```python
from build123d import *

# Parameters (mm, degrees)
F0_R     = 11
F1_DEPTH = 25


with BuildPart() as f1:
    # F0 (on Top) → F1 (new body)
    with BuildSketch(Plane.XY):
        with BuildLine():
            ThreePointArc((12.5, -8.291562), (40, 0), (12.5, 8.291562))
            ThreePointArc((12.5, 8.291562), (10.606602, 10.606602), (8.291562, 12.5))
            ThreePointArc((8.291562, 12.5), (0, 40), (-8.291562, 12.5))
            ThreePointArc((-8.291562, 12.5), (-10.606602, 10.606602), (-12.5, 8.291562))
            ThreePointArc((-12.5, 8.291562), (-40, 0), (-12.5, -8.291562))
            ThreePointArc((-12.5, -8.291562), (-10.606602, -10.606602), (-8.291562, -12.5))
            ThreePointArc((-8.291562, -12.5), (0, -40), (8.291562, -12.5))
            ThreePointArc((8.291562, -12.5), (10.606602, -10.606602), (12.5, -8.291562))
        make_face()
        with Locations((0, -25)):
            Circle(F0_R, mode=Mode.SUBTRACT)
        with Locations((-25, 0)):
            Circle(F0_R, mode=Mode.SUBTRACT)
        Circle(F0_R, mode=Mode.SUBTRACT)
        with Locations((25, 0)):
            Circle(F0_R, mode=Mode.SUBTRACT)
        with Locations((0, 25)):
            Circle(F0_R, mode=Mode.SUBTRACT)
    extrude(amount=F1_DEPTH)


solid = f1.part
```
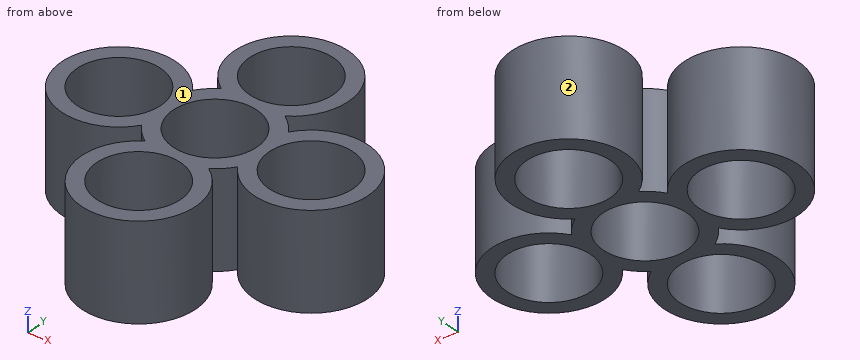
Geometry: final body of the model. Coordinates: model frame, mm. Face numbers are marked on the shaded views. Round coordinates to 2 decimals unless told otherwise and drop trailing zeros. Write each loop counter-clockwise with the first axis right and the second up, starting at its lowest first coordinate (ties: lowest second). Pieces come first, ordered by that corner, then holes. Notation, with made-up numbers: (-20.5, 77.25) -> (29.5, 77.25) arc R18 ccw to (29.5, 101.25) -> close; hole circle Ø8 at (7, 19). An arc over 180 degrees is marked (long way). Use CSV: the item, a comma, the result in double quotes. Start each with the question number.
Q1. Line query: L1, parallel to Y at x = 0, z = 6.5; L2, parallel to X at y = 0.5, z = 11; L3, parallel to Y at x = -25, z = 13.75. Output: solid intervals per line, ascending.
Q2. Section A-A (x = 0). Return loops of the section in (y, z), plus the area to 3 significant figures.
Q3. Section C-C (z = 19). Return loops of the section in (x, y), plus the area to 3 significant figures.
Q4. Section B-B (y = 25). Return loops of the section in (x, z), plus the area to 3 significant figures.
Q5. First-contact query: pin 1 Ø10 at (y, z) = (-21.5, 4.5) entering from +X; pin 2 Ø4 at (x, z) = (-28, 20.5) entering from -Y; pin 3 Ø1.5 at (y, z) = (-13.5, 19.5) entering from +X. Flat tips, straight axial feed; report the tip coordinate or a pass-through.
Q6. Pull-direction query (Y, two-part tool) for the marked faces 1 and 2; classes: pulls with the +Y half, pulls with the -Y half, needs draft (parallel to the pull), parting line crosses it, or undercut.
Result sheet:
1,L1,"-40 to -36, -14 to -11, 11 to 14, 36 to 40"
1,L2,"-39.99 to -35.99, -14.01 to -10.99, 10.99 to 14.01, 35.99 to 39.99"
1,L3,"-15 to -11, 11 to 15"
2,outline,"(-40, 0) -> (-36, 0) -> (-36, 25) -> (-40, 25) -> close; (-14, 0) -> (-11, 0) -> (-11, 25) -> (-14, 25) -> close; (11, 0) -> (14, 0) -> (14, 25) -> (11, 25) -> close; (36, 0) -> (40, 0) -> (40, 25) -> (36, 25) -> close"
2,area,"350 mm²"
3,outline,"(-12.5, -8.29) arc R15 ccw to (-8.29, -12.5) arc R15 ccw (long way) to (8.29, -12.5) arc R15 ccw to (12.5, -8.29) arc R15 ccw (long way) to (12.5, 8.29) arc R15 ccw to (8.29, 12.5) arc R15 ccw (long way) to (-8.29, 12.5) arc R15 ccw to (-12.5, 8.29) arc R15 ccw (long way) to start; hole circle Ø22 at (-25, 0); hole circle Ø22 at (0, -25); hole circle Ø22 at (0, 0); hole circle Ø22 at (0, 25); hole circle Ø22 at (25, 0)"
3,area,"1,410 mm²"
4,outline,"(-15, 0) -> (-11, 0) -> (-11, 25) -> (-15, 25) -> close; (11, 0) -> (15, 0) -> (15, 25) -> (11, 25) -> close"
4,area,"200 mm²"
5,pin 1,"x = 15"
5,pin 2,"y = -14.97"
5,pin 3,"x = 32.9"
6,face 1,"needs draft"
6,face 2,"undercut"
